Geometry check sheet. Reference: the model listing, model coordinates, mm. Coordinates: 2 decimals unless noted, no trailing zeros. Loops run counter-clockwise (first coordinate to the right, second up) from the corner with the lowest first, then second, coordinate; pieces in that order, holes last. Notation, with made-up numbers: (-17.75, -21.75) - (-11.75, -21.75) arc R34 ccw to (-11.75, 14.25) - close; hole circle Ø10 at (-25.75, -12). An arc over 180 degrees is marked (long way). Write item = value, one per line. Start each with the question number.
from build123d import *

# Parameters (mm, degrees)
SKETCH1_W           = 232.41
SKETCH1_H           = 38.1
SKETCH1_R           = 3.175
SKETCH1_R_2         = 6.35
BOSS_EXTRUDE1_DEPTH = 4.7625


with BuildPart() as part:
    # Sketch1 → Boss-Extrude1 (new body)
    with BuildSketch(Plane.XY):
        with Locations((116.205, 19.05)):
            Rectangle(SKETCH1_W, SKETCH1_H)
        with Locations(Location((30.48, 19.05, 0), (0, 0, 180))):
            Circle(SKETCH1_R, mode=Mode.SUBTRACT)
        with Locations(Location((80.01, 19.05, 0), (0, 0, 180))):
            Circle(SKETCH1_R_2, mode=Mode.SUBTRACT)
        with Locations(Location((20.955, 29.21, 0), (0, 0, 180))):
            Circle(SKETCH1_R, mode=Mode.SUBTRACT)
        with Locations(Location((17.78, 8.89, 0), (0, 0, 180))):
            Circle(SKETCH1_R, mode=Mode.SUBTRACT)
        with Locations(Location((214.63, 29.21, 0), (0, 0, 180))):
            Circle(SKETCH1_R, mode=Mode.SUBTRACT)
        with Locations(Location((201.93, 19.05, 0), (0, 0, 180))):
            Circle(SKETCH1_R, mode=Mode.SUBTRACT)
        with Locations(Location((211.455, 8.89, 0), (0, 0, 180))):
            Circle(SKETCH1_R, mode=Mode.SUBTRACT)
        with Locations(Location((54.61, 19.05, 0), (0, 0, 180))):
            Circle(SKETCH1_R_2, mode=Mode.SUBTRACT)
    extrude(amount=BOSS_EXTRUDE1_DEPTH)


solid = part.part
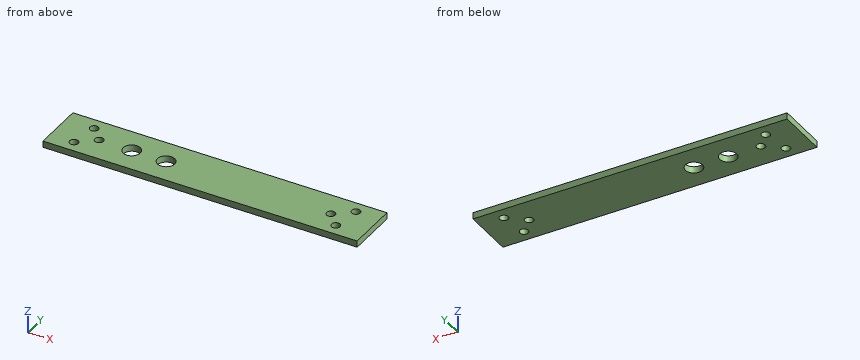
(1) Sectioned sample at B-B on z = 2.8. Count the separate pieces of the cut face and the enclosed holes in it, plus the area to 3 significant figures.
(2) Sectioned sample at C-C on y = 19.05. Enter the section's corners in (x, z) (1 decimal), plus the area to 3 significant figures.
(3) Sectioned sample at A-A on x = 30.48. Enter the section's corners in (y, z) (1 decimal).
(4) Depth check by flat-ended pin: pin 1 (5 mm diameter, centred on x = 20.955, y = 29.21, fed in from -Z). Enter the tip coordinate at first touch or a pass-through.
(5) Sectioned sample at D-D on x = 54.61. Enter the section's corners in (y, z), plus the area to 3 significant figures.
(6) Scan lines: line 1 (X direction, y = 8.89, z = 3.1) (3 decimals); line 2 (X direction, y = 19.05, z = 3.15) (3 decimals); line 3 (X direction, y = 29.21, z = 3.2) (3 decimals). Record each from-to range of solid material in increasing order.
Working result:
q1.separate_pieces = 1
q1.enclosed_holes = 8
q1.area = 8,410 mm2
q2.outline = (0, 0) - (27.3, 0) - (27.3, 4.8) - (0, 4.8) - close; (33.7, 0) - (48.3, 0) - (48.3, 4.8) - (33.7, 4.8) - close; (61, 0) - (73.7, 0) - (73.7, 4.8) - (61, 4.8) - close; (86.4, 0) - (198.8, 0) - (198.8, 4.8) - (86.4, 4.8) - close; (205.1, 0) - (232.4, 0) - (232.4, 4.8) - (205.1, 4.8) - close
q2.area = 925 mm2
q3.outline = (0, 0) - (15.9, 0) - (15.9, 4.8) - (0, 4.8) - close; (22.2, 0) - (38.1, 0) - (38.1, 4.8) - (22.2, 4.8) - close
q4.pin_1 = through
q5.outline = (0, 0) - (12.7, 0) - (12.7, 4.76) - (0, 4.76) - close; (25.4, 0) - (38.1, 0) - (38.1, 4.76) - (25.4, 4.76) - close
q5.area = 121 mm2
q6.line_1 = 0 to 14.605, 20.955 to 208.28, 214.63 to 232.41
q6.line_2 = 0 to 27.305, 33.655 to 48.26, 60.96 to 73.66, 86.36 to 198.755, 205.105 to 232.41
q6.line_3 = 0 to 17.78, 24.13 to 211.455, 217.805 to 232.41
